Read the model definition and answer for the solid it produces. Units are mm, in the model's axes. Face numbers are marked on the shaded views. A direction names the side the tool comes from. Round coordinates to 2 decimals unless told otherwise and drop trailing zeros. Loops run counter-clockwise (first coordinate to the right, second up) from the corner with the lowest first, then second, coordinate; pieces in that order, holes last. Notation, with made-up numbers: M -37,-13 L -2,-13 A10 cw -2,-5 Z; hole C -23.5,40 d3. An arc over 180 degrees is marked long. Write each question's results on one line, items separated by ' | '.
from build123d import *

# Parameters (mm, degrees)
EXTRUDE_1_DEPTH        = 220
CUT_EXTRUDE_1_DEPTH    = 1
PATTERN_LINEAR_3_COUNT = 8
PATTERN_LINEAR_3_PITCH = 25
CUT_EXTRUDE_5_DEPTH    = 9.5
CUT_EXTRUDE_START      = -19.5
CUT_EXTRUDE_6_DEPTH    = 19.5
SKETCH_6_W             = 72.426298227
SKETCH_6_H             = 150
CUT_EXTRUDE_7_DEPTH    = 10


with BuildPart() as part:
    # Эскиз1 → Вытянуть1 (new body)
    with BuildSketch(Plane.XY):
        with BuildLine():
            Line((-17.5, 6.5), (-14.5, 6.5))
            ThreePointArc((-14.5, 6.5), (-13.792893219, 6.207106781), (-13.5, 5.5))
            Line((-13.5, 5.5), (-13.5, 2))
            ThreePointArc((-13.5, 2), (-12.914213562, 0.585786438), (-11.5, 0))
            Line((-11.5, 0), (11.5, 0))
            ThreePointArc((11.5, 0), (12.914213562, 0.585786438), (13.5, 2))
            Line((13.5, 2), (13.5, 5.5))
            ThreePointArc((13.5, 5.5), (13.792893219, 6.207106781), (14.5, 6.5))
            Line((14.5, 6.5), (17.5, 6.5))
            Line((17.5, 6.5), (17.5, 7.5))
            Line((17.5, 7.5), (14.5, 7.5))
            ThreePointArc((14.5, 7.5), (13.085786438, 6.914213562), (12.5, 5.5))
            Line((12.5, 5.5), (12.5, 2))
            ThreePointArc((12.5, 2), (12.207106781, 1.292893219), (11.5, 1))
            Line((11.5, 1), (-11.5, 1))
            ThreePointArc((-11.5, 1), (-12.207106781, 1.292893219), (-12.5, 2))
            Line((-12.5, 2), (-12.5, 5.5))
            ThreePointArc((-12.5, 5.5), (-13.085786438, 6.914213562), (-14.5, 7.5))
            Line((-14.5, 7.5), (-17.5, 7.5))
            Line((-17.5, 7.5), (-17.5, 6.5))
        make_face()
    extrude(amount=EXTRUDE_1_DEPTH)

    # Эскиз2 → Вырез-Вытянуть1 (cut)
    with BuildSketch(Plane(origin=(0, 1, 0), x_dir=(-1, 0, 0), z_dir=(0, 1, 0))):
        with BuildLine():
            Line((3.1, 21.9), (3.1, 13.1))
            ThreePointArc((3.1, 13.1), (0, 10), (-3.1, 13.1))
            Line((-3.1, 13.1), (-3.1, 21.9))
            ThreePointArc((-3.1, 21.9), (0, 25), (3.1, 21.9))
        make_face()
    cut_extrude_1 = extrude(amount=-CUT_EXTRUDE_1_DEPTH, mode=Mode.SUBTRACT)

    # Линейный массив3: Вырез-Вытянуть1 ×8
    with Locations(*[(0, 0, i * PATTERN_LINEAR_3_PITCH) for i in range(1, PATTERN_LINEAR_3_COUNT)]):
        add(cut_extrude_1, mode=Mode.SUBTRACT)

    # Эскиз3 → Вырез-Вытянуть5 (cut)
    with BuildSketch(Plane(origin=(0, 0, 0), x_dir=(-1, 0, 0), z_dir=(0, 0, -1))):
        with BuildLine():
            Line((17.5, 6.5), (17.5, 7.5))
            Line((17.5, 7.5), (14.5, 7.5))
            ThreePointArc((14.5, 7.5), (13.085786438, 6.914213562), (12.5, 5.5))
            Line((12.5, 5.5), (12.5, 2))
            ThreePointArc((12.5, 2), (12.207106781, 1.292893219), (11.5, 1))
            Line((11.5, 1), (-11.5, 1))
            ThreePointArc((-11.5, 1), (-12.207106781, 1.292893219), (-12.5, 2))
            Line((-12.5, 2), (-12.5, 5.5))
            ThreePointArc((-12.5, 5.5), (-13.085786438, 6.914213562), (-14.5, 7.5))
            Line((-14.5, 7.5), (-17.5, 7.5))
            Line((-17.5, 7.5), (-17.5, 6.5))
            Line((-17.5, 6.5), (-14.5, 6.5))
            ThreePointArc((-14.5, 6.5), (-13.792893219, 6.207106781), (-13.5, 5.5))
            Line((-13.5, 5.5), (-13.5, 2))
            ThreePointArc((-13.5, 2), (-12.914213562, 0.585786438), (-11.5, 0))
            Line((-11.5, 0), (11.5, 0))
            ThreePointArc((11.5, 0), (12.914213562, 0.585786438), (13.5, 2))
            Line((13.5, 2), (13.5, 5.5))
            ThreePointArc((13.5, 5.5), (13.792893219, 6.207106781), (14.5, 6.5))
            Line((14.5, 6.5), (17.5, 6.5))
        make_face()
    extrude(amount=-CUT_EXTRUDE_5_DEPTH, mode=Mode.SUBTRACT)

    # Эскиз5 → Вырез-Вытянуть6 (cut)
    with BuildSketch(Plane.XY.offset(220).offset(CUT_EXTRUDE_START)):
        with BuildLine():
            Line((-17.5, 7.5), (-17.5, 6.5))
            Line((-17.5, 6.5), (-14.5, 6.5))
            ThreePointArc((-14.5, 6.5), (-13.792893219, 6.207106781), (-13.5, 5.5))
            Line((-13.5, 5.5), (-13.5, 2))
            ThreePointArc((-13.5, 2), (-12.914213562, 0.585786438), (-11.5, 0))
            Line((-11.5, 0), (11.5, 0))
            ThreePointArc((11.5, 0), (12.914213562, 0.585786438), (13.5, 2))
            Line((13.5, 2), (13.5, 5.5))
            ThreePointArc((13.5, 5.5), (13.792893219, 6.207106781), (14.5, 6.5))
            Line((14.5, 6.5), (17.5, 6.5))
            Line((17.5, 6.5), (17.5, 7.5))
            Line((17.5, 7.5), (14.5, 7.5))
            ThreePointArc((14.5, 7.5), (13.085786438, 6.914213562), (12.5, 5.5))
            Line((12.5, 5.5), (12.5, 2))
            ThreePointArc((12.5, 2), (12.207106781, 1.292893219), (11.5, 1))
            Line((11.5, 1), (-11.5, 1))
            ThreePointArc((-11.5, 1), (-12.207106781, 1.292893219), (-12.5, 2))
            Line((-12.5, 2), (-12.5, 5.5))
            ThreePointArc((-12.5, 5.5), (-13.085786438, 6.914213562), (-14.5, 7.5))
            Line((-14.5, 7.5), (-17.5, 7.5))
        make_face()
    extrude(amount=CUT_EXTRUDE_6_DEPTH, mode=Mode.SUBTRACT)

    # Эскиз6 → Вырез-Вытянуть7 (cut)
    with BuildSketch(Plane.XZ):
        with Locations((4.055872701, 59.5)):
            Rectangle(SKETCH_6_W, SKETCH_6_H)
    extrude(amount=-CUT_EXTRUDE_7_DEPTH, mode=Mode.SUBTRACT)


solid = part.part
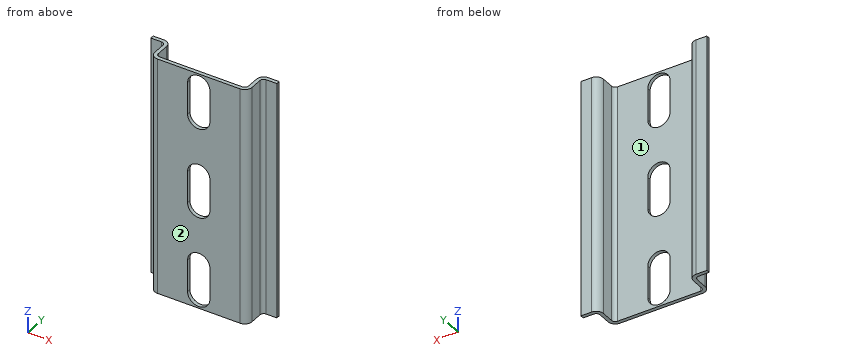
Item 1: Straight lines are drawn through the part: line 1 (X direction, y = 2.75, z = 167); line 2 (Y direction, x = 5, z = 172); line 3 (X direction, y = 6.75, z = 196.5). For each, find the intervals that lie inside material, in ascending order.
Outcome:
line 1: x = -13.5 to -12.5, 12.5 to 13.5 | line 2: y = 0 to 1 | line 3: x = -17.5 to -12.94, 12.94 to 17.5
Item 2: The part is cut by section D-D (z = 153). Determine the outline of the cut face in (x, y), plus the area to 3 significant figures.
Outcome:
outline: M -17.5,6.5 L -14.5,6.5 A1 cw -13.5,5.5 L -13.5,2 A2 ccw -11.5,0 L 11.5,0 A2 ccw 13.5,2 L 13.5,5.5 A1 cw 14.5,6.5 L 17.5,6.5 L 17.5,7.5 L 14.5,7.5 A2 ccw 12.5,5.5 L 12.5,2 A1 cw 11.5,1 L -11.5,1 A1 cw -12.5,2 L -12.5,5.5 A2 ccw -14.5,7.5 L -17.5,7.5 Z | area: 45.4 mm2
Item 3: The part is cut by section B-B (z = 166). Determine the outline of the cut face in (x, y).
Outcome:
outline: M -17.5,6.5 L -14.5,6.5 A1 cw -13.5,5.5 L -13.5,2 A2 ccw -11.5,0 L -3.1,0 L -3.1,1 L -11.5,1 A1 cw -12.5,2 L -12.5,5.5 A2 ccw -14.5,7.5 L -17.5,7.5 Z; M 3.1,0 L 11.5,0 A2 ccw 13.5,2 L 13.5,5.5 A1 cw 14.5,6.5 L 17.5,6.5 L 17.5,7.5 L 14.5,7.5 A2 ccw 12.5,5.5 L 12.5,2 A1 cw 11.5,1 L 3.1,1 Z
Item 4: The part is cut by section A-A (y = 3.75). Determine the outline of the cut face in (x, z).
Outcome:
outline: M -13.5,134.5 L -12.5,134.5 L -12.5,200.5 L -13.5,200.5 Z; M 12.5,134.5 L 13.5,134.5 L 13.5,200.5 L 12.5,200.5 Z
Item 5: Flat-ended cylindrical pins translate along their axes: pin 1 (10 mm diameter, centred on x = -1.5, z = 144.5, fed in from +Y); pin 2 (0.5 mm diameter, centred on y = 0.5, z = 193, fed in from -X); pin 3 (0.5 mm diameter, centred on y = 0.5, z = 167, fed in from +X); pin 4 (8 mm diameter, centred on x = -4, z = 176.5, fed in from -Y). Find the tip coordinate at first contact, or state that the pin passes through.
Outcome:
pin 1: stops at y = 1 | pin 2: stops at x = -13.06 | pin 3: stops at x = 13.06 | pin 4: stops at y = 0
Item 6: For the marked faces 1 and 2, determine the directions among +Z, -Z, +X, -X, +Y, -Y from which every point of the face is accessible in a straight line to the end or side of a thin tool.
Outcome:
face 1: +Z, -Z, +Y | face 2: +Z, -Z, +X, -X, -Y
Item 7: The part is cut by section C-C (x = 0). Determine the outline of the cut face in (y, z).
Outcome:
outline: M 0,134.5 L 1,134.5 L 1,135 L 0,135 Z; M 0,150 L 1,150 L 1,160 L 0,160 Z; M 0,175 L 1,175 L 1,185 L 0,185 Z; M 0,200 L 1,200 L 1,200.5 L 0,200.5 Z
